from build123d import *

# Parameters (mm, degrees)
F1_DEPTH = 280
F3_DEPTH = 280


with BuildPart() as f1:
    # F0 (on Front) → F1 (new body)
    with BuildSketch(Plane.XZ):
        with BuildLine():
            Line((-32.75, 3.5), (-33, 18.5))
            Line((-33, 18.5), (-34.5, 18.5))
            Line((-34.5, 18.5), (-34.722757, 3.5))
            Line((-34.722757, 3.5), (-34.722757, -10.5))
            Line((-34.722757, -10.5), (-27.722757, -10.5))
            Line((-27.722757, -10.5), (-27.722757, -5.971823))
            Line((-27.722757, -5.971823), (-28.722757, -5.971823))
            Line((-28.722757, -5.971823), (-28.722757, -7.471823))
            Line((-28.722757, -7.471823), (-30.722757, -7.471823))
            Line((-30.722757, -7.471823), (-30.722757, -5.232051))
            Line((-30.722757, -5.232051), (-27.722757, -3.5))
            Line((-27.722757, -3.5), (-25.722757, -3.5))
            Line((-25.722757, -3.5), (-25.722757, -8.5))
            Line((-25.722757, -8.5), (-24.222757, -8.5))
            Line((-24.222757, -8.5), (-24.222757, -3.5))
            Line((-24.222757, -3.5), (-10.465052, -3.5))
            Line((-10.465052, -3.5), (-12.465052, -1.821801))
            Line((-12.465052, -1.821801), (-12.465052, -0.821801))
            ThreePointArc((-12.465052, -0.821801), (-11.465052, 0.178199), (-10.465052, -0.821801))
            Line((-10.465052, -0.821801), (-10.465052, -1.221801))
            Line((-10.465052, -1.221801), (-7.75, -3.5))
            Line((-7.75, -3.5), (0, -3.5))
            Line((0, -3.5), (0, 38.5))
            Line((0, 38.5), (-0.75, 38.5))
            Line((-0.75, 38.5), (-1, 3.5))
            Line((-1, 3.5), (-5.75, 3.5))
            Line((-5.75, 3.5), (-6, 33.5))
            Line((-6, 33.5), (-7.5, 33.5))
            Line((-7.5, 33.5), (-7.75, 3.5))
            Line((-7.75, 3.5), (-12.75, 3.5))
            Line((-12.75, 3.5), (-12.75, 28.5))
            Line((-12.75, 28.5), (-14.25, 28.5))
            Line((-14.25, 28.5), (-14.5, 3.5))
            Line((-14.5, 3.5), (-19.25, 3.5))
            Line((-19.25, 3.5), (-19.5, 23.5))
            Line((-19.5, 23.5), (-21, 23.5))
            Line((-21, 23.5), (-21.238413, 3.5))
            Line((-21.238413, 3.5), (-26.014383, 3.5))
            Line((-26.014383, 3.5), (-26.25, 21))
            Line((-26.25, 21), (-27.75, 21))
            Line((-27.75, 21), (-28, 3.5))
            Line((-28, 3.5), (-32.75, 3.5))
        make_face()
    extrude(amount=F1_DEPTH)

    # F2 (on face) → F3 (join)
    with BuildSketch(Plane.XZ.offset(280)):
        Polygon((-34.722757, -10.5), (-34.722757, -8.503925), (-39.222757, -8.503925), (-45.113872, -2.987565), (-46.174532, -4.048225), (-39.722757, -10.5), align=None)
        Polygon((-46.174532, 7.951775), (-39.722757, 1.5), (-34.722757, 1.5), (-34.722757, 3.496075), (-39.222757, 3.496075), (-45.113872, 9.012435), align=None)
    extrude(amount=-F3_DEPTH)

    # F4: F1 across face


with BuildPart() as f1_1:
    add(f1.part)
    add(f1.part.mirror(Plane(origin=(0, -140, 17.5), x_dir=(0, 1, 0), z_dir=(1, 0, 0))))


solid = f1_1.part
Check sheet for the modelled part. Datum: model origin and axes. Units: mm. A direction names the side the tool comes from. Round coordinates to 2 decimals unless told otherwise and drop trailing zeros. One line per question, with ' | ' between items. Start each with the question number.
Item 1: Set-up check for faces 1 (the face through (37, -142, -8.504)), 2 (the face through (3, -138, 3.5)), 3 (the face through (-24.223, -138, -6)): record each of +Z, -Z, +X, -X, +Y, -Y from which the full face is reachable in a straight line by a thin tool's end or side.
Item 2: Gauge pin test, flat ends, axial feed: pin 1 Ø3 at (y, z) = (-163, 0.5) entering from +X; pin 2 Ø2 at (x, y) = (37, -133.5) entering from +Z; pin 3 Ø1.1 at (y, z) = (-193.5, -1.5) entering from -X; pin 4 Ø2 at (x, z) = (3.5, 25) entering from +Y. Record the tip position at first contact, or that the pin passes through.
Item 3: Release check for a two-part mould opening along X. For faces 4 (the face through (0, -280, 9)), 5 (the face through (-30, -138, 3.5)), 6 (the face through (42.99, -141.96, -7.23)) record: released by +X, released by -X, zero draft, split by the parting line, or undercut.
Item 4: Scan lines: probe 1 along X at (y, z) = (-40.5, 31.5); probe 2 along Z at (x, y) = (-38, -106); probe 3 along X at (y, z) = (-237, 27.5). Record each from-to range of solid material in increasing order.
Worked out:
1) face 1: +Y, -Y | face 2: +Z, +Y, -Y | face 3: -Z, +Y, -Y
2) pin 1: x = 40.22 | pin 2: z = 3.5 | pin 3: x = -34.72 | pin 4: through
3) face 4: zero draft | face 5: undercut | face 6: released by +X
4) probe 1: -7.52 to -5.98, -0.8 to 0.8, 5.98 to 7.52 | probe 2: -10.5 to -8.5, 1.5 to 3.5 | probe 3: -14.26 to -12.75, -7.55 to -5.95, -0.83 to 0.83, 5.95 to 7.55, 12.75 to 14.26
